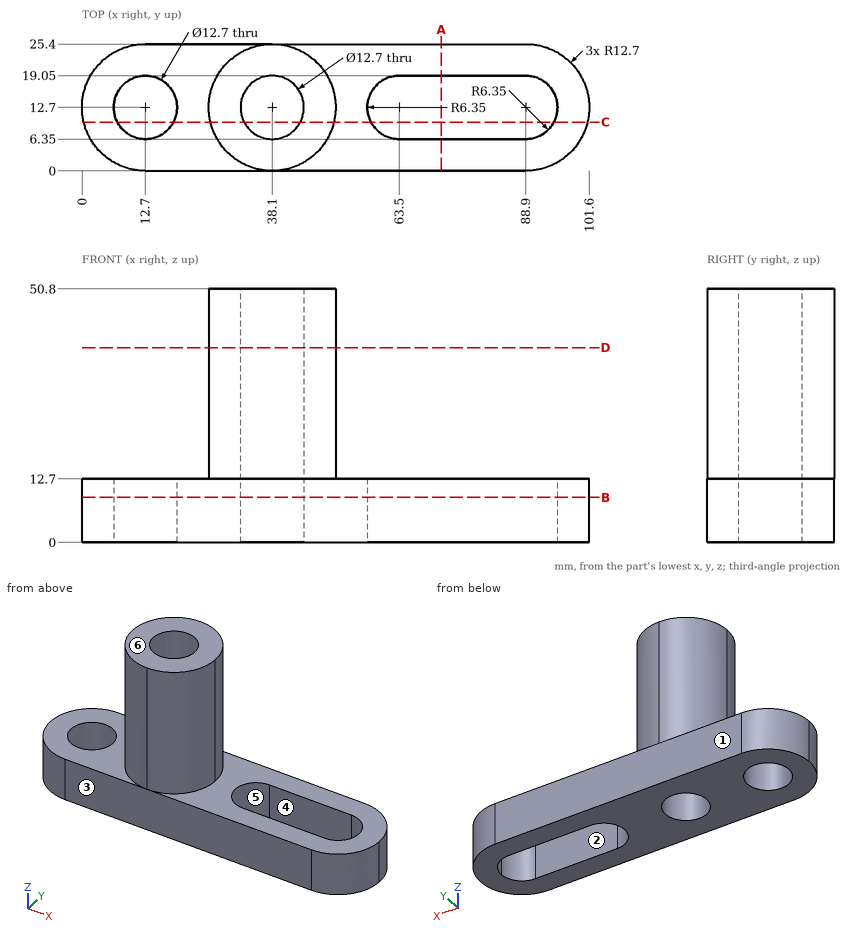
Here's the drawing with two shaded views (mm, measured from the low corner). I have some questions. A direction names the side the tool comes from. Coordinates: 2 decimals unless noted, no trailing zeros. Order: outer loops, then holes, each group sorted by start corner. A loop starts at its lowest first (then second) coordinate and runs counter-clockwise, first axis right, second up.
Item 1: If we section it at A-A on x = 72: List the corners of the cut face in (y, z) for me, plus the area to 3 significant figures.
Result sheet:
outline: (0, 0) - (6.35, 0) - (6.35, 12.7) - (0, 12.7) - close; (19.05, 0) - (25.4, 0) - (25.4, 12.7) - (19.05, 12.7) - close
area: 161 mm2
Item 2: I need wall thicknesses on line 1 (Y direction, x = 38, z = 15); line 2 (X direction, y = 8.5, z = 5); line 3 (Z direction, x = 18, y = 8.25). Which ranges of each line are inside material? Lowest first, please.
Result sheet:
line 1: y = 0 to 6.35, 19.05 to 25.4
line 2: x = 0.71 to 7.94, 17.46 to 33.34, 42.86 to 58.74, 93.66 to 100.89
line 3: z = 0 to 12.7
Item 3: If we mould it in two halves opening along Y, with no side actions, what happens to the marked faces 3, 4, 5 and 6? For each: +Y half, -Y half, draft (parallel to the pull), parting line (faces both ways), or undercut.
Result sheet:
face 3: -Y half
face 4: undercut
face 5: undercut
face 6: draft
Item 4: For the marked faces 1 and 2, which set-ups out of +Z, -Z, +X, -X, +Y, -Y let a thin tool reach every point of the face, with its end or its side?
Result sheet:
face 1: +Z, -Z, +X, -X, +Y
face 2: +Z, -Z
Item 5: If we section it at B-B on z = 9: List the corners of the cut face in (x, y) for me.
Result sheet:
outline: (12.7, 0) - (88.9, 0) arc R12.7 ccw to (88.9, 25.4) - (12.7, 25.4) arc R12.7 ccw to start; hole circle Ø12.7 at (12.7, 12.7); hole circle Ø12.7 at (38.1, 12.7); hole (63.5, 6.35) - (88.9, 6.35) arc R6.35 ccw to (88.9, 19.05) - (63.5, 19.05) arc R6.35 ccw to start
Item 6: For P1, Ø1, axis at x = 53, y = 21.5, coming from the -Z side; P2, Ø1.5, axis at y = 23, z = 12, coming from the -X side; P3, Ø8, axis at y = 12.5, z = 22, coming from the -X side; P4, Ø8, axis at x = 50.5, z = 39, coming from the +Y side, each with a flat end and sliding along its axis, tell me the tip position at first contact or that it passes through.
Result sheet:
P1: stops at z = 0
P2: stops at x = 4.33
P3: stops at x = 25.4
P4: stops at y = 22.23
Item 7: If we section it at D-D on z = 39: List the corners of the cut face in (x, y) for me, plus the area to 3 significant figures.
Result sheet:
outline: circle Ø25.4 at (38.1, 12.7); hole circle Ø12.7 at (38.1, 12.7)
area: 380 mm2
Item 8: If we section it at C-C on y = 9.75: List the corners of the cut face in (x, z) for me, plus the area to 3 significant figures.
Result sheet:
outline: (0.35, 0) - (7.08, 0) - (7.08, 12.7) - (0.35, 12.7) - close; (18.32, 0) - (32.48, 0) - (32.48, 50.8) - (25.75, 50.8) - (25.75, 12.7) - (18.32, 12.7) - close; (43.72, 0) - (57.88, 0) - (57.88, 12.7) - (50.45, 12.7) - (50.45, 50.8) - (43.72, 50.8) - close; (94.52, 0) - (101.25, 0) - (101.25, 12.7) - (94.52, 12.7) - close
area: 1,040 mm2
